CAD build for the part. Positions are in the model's coordinates, mm. Face numbers are marked on the shaded views. A direction names the side the tool comes from. Coordinates: 2 decimals unless noted, no trailing zeros. Order: outer loops, then holes, each group sorted by start corner. A loop starts at its lowest first (then second) coordinate and runs counter-clockwise, first axis right, second up.
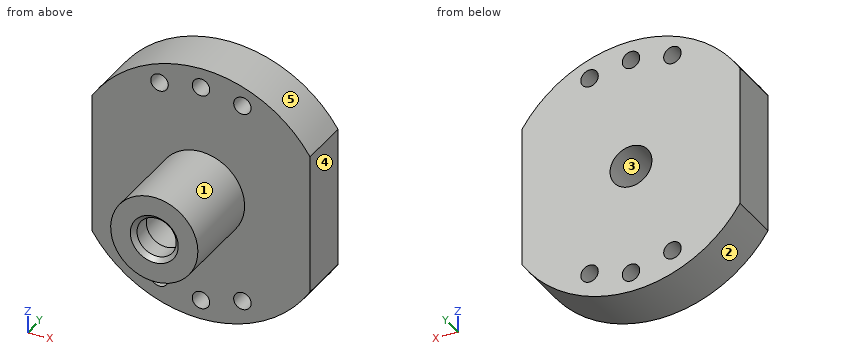
from build123d import *

# Parameters (mm, degrees)
SKETCH1_R           = 2
BOSS_EXTRUDE1_DEPTH = 12
SKETCH2_R           = 4.8
CUT_EXTRUDE1_DEPTH  = 74.394724572
CHAMFER1_SIZE       = 1


with BuildPart() as part:
    # Sketch1 → Boss-Extrude1 (new body)
    # profile 1 of 2: a face of its own
    with BuildSketch(Plane.XZ.offset(18)):
        with BuildLine():
            Line((-23.453342414, -21.61684273), (-23.453342414, -53.703414688))
            ThreePointArc((-23.453342414, -53.703414688), (1.546657586, -67.365128709), (26.546657586, -53.703414688))
            Line((26.546657586, -53.703414688), (26.546657586, -21.61684273))
            ThreePointArc((26.546657586, -21.61684273), (1.546657586, -7.955128709), (-23.453342414, -21.61684273))
        make_face()
        with Locations(Location((-7.953342414, -60.376565813, 0), (0, 0, 270))):
            Circle(SKETCH1_R, mode=Mode.SUBTRACT)
        with BuildLine():
            ThreePointArc((16.671348492, -51.125128709), (1.546657586, -57.910128709), (-13.57803332, -51.125128709))
            Line((-13.57803332, -51.125128709), (-13.57803332, -45.660128709))
            Line((-13.57803332, -45.660128709), (-17.056097586, -45.660128709))
            ThreePointArc((-17.056097586, -45.660128709), (-18.703342414, -37.660128709), (-17.056097586, -29.660128709))
            Line((-17.056097586, -29.660128709), (-13.57803332, -29.660128709))
            Line((-13.57803332, -29.660128709), (-13.57803332, -24.195128709))
            ThreePointArc((-13.57803332, -24.195128709), (1.546657586, -17.410128709), (16.671348492, -24.195128709))
            Line((16.671348492, -24.195128709), (16.671348492, -29.660128709))
            Line((16.671348492, -29.660128709), (20.149412759, -29.660128709))
            Line((20.149412759, -29.660128709), (20.149412759, -32.660128709))
            Line((20.149412759, -32.660128709), (16.671348492, -32.660128709))
            Line((16.671348492, -32.660128709), (16.671348492, -42.660128709))
            Line((16.671348492, -42.660128709), (20.149412759, -42.660128709))
            Line((20.149412759, -42.660128709), (20.149412759, -45.660128709))
            Line((20.149412759, -45.660128709), (16.671348492, -45.660128709))
            Line((16.671348492, -45.660128709), (16.671348492, -51.125128709))
        make_face(mode=Mode.SUBTRACT)
        with Locations(Location((1.546657586, -62.910128709, 0), (0, 0, 270))):
            Circle(SKETCH1_R, mode=Mode.SUBTRACT)
        with Locations(Location((11.046657586, -60.376565813, 0), (0, 0, 270))):
            Circle(SKETCH1_R, mode=Mode.SUBTRACT)
        with Locations(Location((-7.953342414, -14.026565813, 0), (0, 0, 270))):
            Circle(SKETCH1_R, mode=Mode.SUBTRACT)
        with Locations(Location((11.046657586, -14.026565813, 0), (0, 0, 270))):
            Circle(SKETCH1_R, mode=Mode.SUBTRACT)
        with Locations(Location((1.546657586, -12.410128709, 0), (0, 0, 270))):
            Circle(SKETCH1_R, mode=Mode.SUBTRACT)
    # profile 2 of 2: a face of its own
    with BuildSketch(Plane.XZ.offset(18)):
        with BuildLine():
            Line((-13.57803332, -51.125128709), (-13.57803332, -45.660128709))
            Line((-13.57803332, -45.660128709), (-17.056097586, -45.660128709))
            ThreePointArc((-17.056097586, -45.660128709), (-18.703342414, -37.660128709), (-17.056097586, -29.660128709))
            Line((-17.056097586, -29.660128709), (-13.57803332, -29.660128709))
            Line((-13.57803332, -29.660128709), (-13.57803332, -24.195128709))
            ThreePointArc((-13.57803332, -24.195128709), (1.546657586, -17.410128709), (16.671348492, -24.195128709))
            Line((16.671348492, -24.195128709), (16.671348492, -29.660128709))
            Line((16.671348492, -29.660128709), (20.149412759, -29.660128709))
            Line((20.149412759, -29.660128709), (20.149412759, -32.660128709))
            Line((20.149412759, -32.660128709), (16.671348492, -32.660128709))
            Line((16.671348492, -32.660128709), (16.671348492, -42.660128709))
            Line((16.671348492, -42.660128709), (20.149412759, -42.660128709))
            Line((20.149412759, -42.660128709), (20.149412759, -45.660128709))
            Line((20.149412759, -45.660128709), (16.671348492, -45.660128709))
            Line((16.671348492, -45.660128709), (16.671348492, -51.125128709))
            ThreePointArc((16.671348492, -51.125128709), (1.546657586, -57.910128709), (-13.57803332, -51.125128709))
        make_face()
    extrude(amount=BOSS_EXTRUDE1_DEPTH)

    # Sketch2 → Cut-Extrude1 (cut, through all)
    with BuildSketch(Plane.XZ.offset(30)):
        with Locations(Location((1.546657586, -37.660128709, 0), (0, 0, 270))):
            Circle(SKETCH2_R)
    extrude(amount=-CUT_EXTRUDE1_DEPTH, mode=Mode.SUBTRACT)

    # Sketch3 → Revolve1 (revolve)
    with BuildSketch(Plane(origin=(1.546657586, 0, 0), x_dir=(0, 0, -1), z_dir=(1, 0, 0))):
        Polygon((27.660128709, -50), (27.660128709, -30), (32.860128709, -30), (32.860128709, -45), (33.160128709, -45), (33.160128709, -50), align=None)
    revolve(axis=Axis((1.546657586, -30, -37.660128709), (0, -1, 0)))

    # Chamfer1
    chamfer1_edges = [part.edges().sort_by_distance(p)[0] for p in [
        (1.546657586, -50, -42.160128709),
    ]]
    chamfer(chamfer1_edges, length=CHAMFER1_SIZE)


solid = part.part
1) Slice it at C-C (z = -19). List the corners of the cut face in (x, y), plus the area to 3 significant figures.
2) Slice it at B-B (x = 2.5). Give the number of separate pieces and of enclosed holes in the cut face, plus the area to 3 significant figures.
3) Which spindle directions (+Z, -Z, +X, -X, +Y, -Y) get a long thin tool onto all of the face, cutting with end or side? Do the marked faces 1 and 2. Say none if no direction does.
4) Drill centre lines: probe 1 along X at (y, z) = (-29.5, -15); probe 2 along Y at (x, z) = (-2.5, -28); probe 3 along Z at (x, y) = (-1, -27.5). Where is each one in solid material? Low to high.
5) Slice it at A-A (y = -22). List the corners of the cut face in (x, z) (3 decimals), plus the area to 3 significant figures.
6) Pin check, flat tips, straight feed: P1, Ø4.5, axis at x = -7.95, z = -60.38, coming from the -Y side; P2, Ø12, axis at y = -32.5, z = -17.5, coming from the +X side; P3, Ø3, axis at y = -42.5, z = -30, coming from the +X side; P4, Ø6, axis at x = 1.55, z = -37.66, coming from the -Y side. Stop position of each tip, or through.
7) Two-plate mould, pull along Z, no slides. Class the marked faces 3, 4 and 5: released by +Z, released by -Z, zero draft, split by the parting line, or undercut.
8) Slice it at D-D (y = -41). List the corners of the cut face in (x, z), plus the area to 3 significant figures.
Worked out:
1. outline: (-21.57, -30) - (24.66, -30) - (24.66, -18) - (-21.57, -18) - close
1. area: 555 mm2
2. separate pieces: 4
2. enclosed holes: 0
2. area: 727 mm2
3. face 1: -Y
3. face 2: -Z, +Y, -Y
4. probe 1: x = -17.66 to -9.7, -6.21 to 9.3, 12.79 to 20.75
4. probe 2: y = -30 to -18
4. probe 3: z = -67.26 to -41.73, -33.59 to -8.06
5. outline: (-23.453, -53.703) arc R29.705 ccw to (26.547, -53.703) - (26.547, -21.617) arc R29.705 ccw to (-23.453, -21.617) - close; hole circle Ø4 at (-7.953, -60.377); hole circle Ø4 at (-7.953, -14.027); hole circle Ø9.6 at (1.547, -37.66); hole circle Ø4 at (1.547, -62.91); hole circle Ø4 at (1.547, -12.41); hole circle Ø4 at (11.047, -60.377); hole circle Ø4 at (11.047, -14.027)
5. area: 2,420 mm2
6. P1: stops at y = -30
6. P2: stops at x = 26.55
6. P3: stops at x = 9.42
6. P4: passes through
7. face 3: undercut
7. face 4: zero draft
7. face 5: released by +Z
8. outline: circle Ø20 at (1.55, -37.66); hole circle Ø9.6 at (1.55, -37.66)
8. area: 242 mm2
